Geometry check sheet. Reference: the model listing, model coordinates, mm. Coordinates: 2 decimals unless noted, no trailing zeros. Order: outer loops, then holes, each group sorted by start corner. A loop starts at its lowest first (then second) coordinate and runs counter-clockwise, first axis right, second up. Notation, with made-up numbers: (52, 24) - (83, 24) arc R21 cw to (83, 40) - close; hole circle Ø7 at (-10, -14.5). An arc over 180 degrees is marked (long way). Return JSON: item names as keys, results as strings. Group by question number.
Item 1: Draft check along Y on faces 1 (the cylindrical face through (-8.881, 5.458, 13.163)), 2 (the cylindrical face through (-8.881, -11.172, 7.123)). Enter one of: pulls with the +Y half, pulls with the -Y half, needs draft (parallel to the pull), parting line crosses it, or undercut.
Item 2: Section check C-C on x = -7.25. Enter the section's corners in (y, z), then the cut area to 3 significant figures.
Item 3: Gauge pin test, flat ends, axial feed: pin 1 (8 mm diameter, centred on x = -3.5, y = 1.5, fed in from +Z); pin 2 (3 mm diameter, centred on x = -12.5, z = -9, fed in from +Y); pin 3 (4 mm diameter, centred on x = -7, y = 10, fed in from -Z); pin 4 (1 mm diameter, centred on x = -5, z = 3, fed in from -Y). Record the tip position at first contact, or that the pin passes through.
Item 4: Scan lines: probe 1 along Z at (x, y) = (-8, 0); probe 2 along Y at (x, z) = (-13, -5). Record each from-to range of solid material in increasing order.
from build123d import *

# Parameters (mm, degrees)
F0_W = 18
F0_H = 1
F2_R = 0.49999
F3_R = 0.49999


# Not quite as in the source:
# - a fillet or chamfer is up to 0.001 mm smaller than in the source, because OpenCascade refuses the exact size


with BuildPart() as f1:
    # F0 (on Front) → F1 (revolve)
    with BuildSketch(Plane.XZ):
        with Locations((-9, 13.75)):
            Rectangle(F0_W, F0_H)
    revolve(axis=Axis((-8.2086159056, 0, 0), (1, 0, 0)))

    # F2 (radius 0.5 in the source; OpenCascade refuses exactly that, so slightly less here)
    f2_edges = [f1.edges().sort_by_distance(p)[0] for p in [
        (0, 0, -13.25),
        (0, 0, -14.25),
    ]]
    fillet(f2_edges, radius=F2_R)

    # F3 (radius 0.5 in the source; OpenCascade refuses exactly that, so slightly less here)
    f3_edges = [f1.edges().sort_by_distance(p)[0] for p in [
        (-18, 0, -14.25),
        (-18, 0, -13.25),
    ]]
    fillet(f3_edges, radius=F3_R)


solid = f1.part
Computed:
{
 "1": {"face 1": "parting line crosses it", "face 2": "undercut"},
 "2": {"outline": "circle Ø28.5 at (0, 0); hole circle Ø26.5 at (0, 0)", "area": "86.4 mm²"},
 "3": {"pin 1": "stops at z = 14.25", "pin 2": "stops at y = 12.12", "pin 3": "stops at z = -11.79", "pin 4": "stops at y = -14.03"},
 "4": {"probe 1": "z = -14.25 to -13.25, 13.25 to 14.25", "probe 2": "y = -13.34 to -12.27, 12.27 to 13.34"}
}
